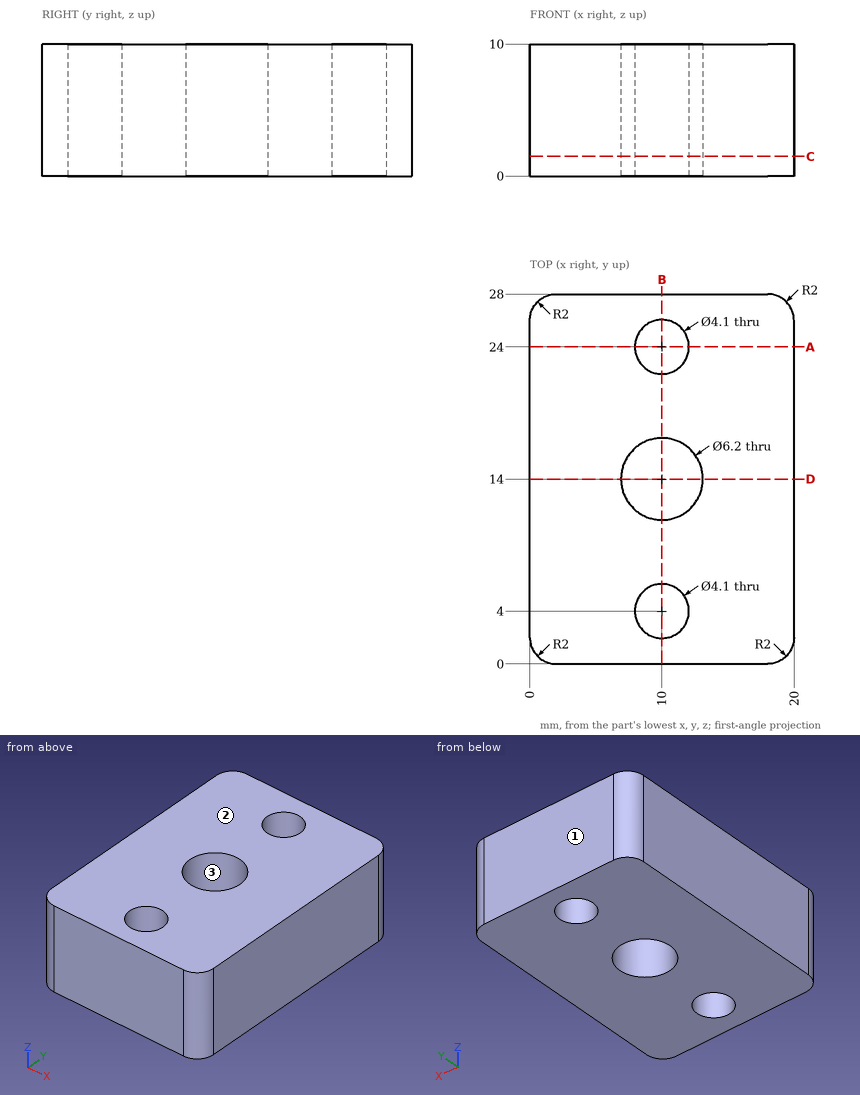
Geometry: see drawing. Coordinates: mm, zero at the bounding-box minimum. Round coordinates to 2 decimals unless told otherwise and drop trailing zeros. Order: outer loops, then holes, each group sorted by start corner. A loop starts at its lowest first (then second) coordinate and runs counter-clockwise, first axis right, second up. Notation, with made-up numbers: (-7.5, 54) -> (36.5, 54) arc R11 cw to (36.5, 71) -> close; hole circle Ø7 at (7, 41.25). An arc over 180 degrees is marked (long way). Write each question's results on one line, items separated by ' | '.
Q1. Section query B-B (x = 10). Output: boundary loops of the cut face in (y, z).
Response values:
outline: (0, 0) -> (1.95, 0) -> (1.95, 10) -> (0, 10) -> close; (6.05, 0) -> (10.9, 0) -> (10.9, 10) -> (6.05, 10) -> close; (17.1, 0) -> (21.95, 0) -> (21.95, 10) -> (17.1, 10) -> close; (26.05, 0) -> (28, 0) -> (28, 10) -> (26.05, 10) -> close
Q2. Pull-direction query (Y, two-part tool) for the marked faces 1, 2 and 3; classes: released by +Y, released by -Y, zero draft, split by the parting line, or undercut.
Response values:
face 1: released by +Y | face 2: zero draft | face 3: undercut
Q3. Section query D-D (y = 14). Output: boundary loops of the cut face in (x, z).
Response values:
outline: (0, 0) -> (6.9, 0) -> (6.9, 10) -> (0, 10) -> close; (13.1, 0) -> (20, 0) -> (20, 10) -> (13.1, 10) -> close
Q4. Ray query, line 1 along Y through (x, z) = (10, 2.5); line 2 along Y through (x, z) = (8.5, 8.25); line 3 along X through (y, z) = (16.25, 3.5). Return the intervals inside material, ascending.
Response values:
line 1: 0 to 1.95, 6.05 to 10.9, 17.1 to 21.95, 26.05 to 28 | line 2: 0 to 2.6, 5.4 to 11.29, 16.71 to 22.6, 25.4 to 28 | line 3: 0 to 7.87, 12.13 to 20
Q5. Section query A-A (y = 24). Output: boundary loops of the cut face in (x, z).
Response values:
outline: (0, 0) -> (7.95, 0) -> (7.95, 10) -> (0, 10) -> close; (12.05, 0) -> (20, 0) -> (20, 10) -> (12.05, 10) -> close
Q6. Section query C-C (z = 1.5). Output: boundary loops of the cut face in (x, y).
Response values:
outline: (0, 2) arc R2 ccw to (2, 0) -> (18, 0) arc R2 ccw to (20, 2) -> (20, 26) arc R2 ccw to (18, 28) -> (2, 28) arc R2 ccw to (0, 26) -> close; hole circle Ø6.2 at (10, 14); hole circle Ø4.1 at (10, 4); hole circle Ø4.1 at (10, 24)
Q7. Pin query (flat end, axial travel): pin 1 Ø4.5 at (x, y) = (10, 4) entering from -Z. Return the tip coordinate at first contact, or that it passes through.
Response values:
pin 1: z = 0
